```python
from build123d import *

# Parameters (mm, degrees)
BOSS_EXTRUDE1_DEPTH   = 9
BOSS_EXTRUDE1_2_DEPTH = 9
SKETCH1_3_W           = 6
SKETCH1_3_H           = 30
BOSS_EXTRUDE2_DEPTH   = 28
BOSS_EXTRUDE2_2_DEPTH = 28
SKETCH1_4_W           = 4
SKETCH1_4_H           = 7
BOSS_EXTRUDE3_DEPTH   = 40
BOSS_EXTRUDE3_2_DEPTH = 40
BOSS_EXTRUDE3_3_DEPTH = 40
BOSS_EXTRUDE3_4_DEPTH = 40
SKETCH1_5_W           = 10
SKETCH1_5_H           = 3
BOSS_EXTRUDE4_DEPTH   = 35.5
BOSS_EXTRUDE4_2_DEPTH = 35.5
SKETCH1_6_W           = 120
SKETCH1_6_H           = 60
BOSS_EXTRUDE5_DEPTH   = 2
SKETCH1_8_W           = 28.6
SKETCH1_8_H           = 57
SKETCH1_8_W_2         = 22.6
SKETCH1_8_H_2         = 51
BOSS_EXTRUDE6_DEPTH   = 9
SKETCH1_9_W           = 22.6
SKETCH1_9_H           = 0.6
BOSS_EXTRUDE7_DEPTH   = 9
SKETCH2_W             = 6
SKETCH2_H             = 3.75
BOSS_EXTRUDE8_DEPTH   = 13
BOSS_EXTRUDE9_DEPTH   = 3
SKETCH3_5_R           = 1.5
BOSS_EXTRUDE11_DEPTH  = 8
SKETCH4_R             = 4.5
SKETCH4_R_2           = 1.5
BOSS_EXTRUDE13_DEPTH  = 4
SKETCH4_4_R           = 1.5
CUT_EXTRUDE2_DEPTH    = 4
SKETCH5_R             = 4.5
SKETCH5_R_2           = 1.5
BOSS_EXTRUDE14_DEPTH  = 4
SKETCH5_2_R           = 1.5
CUT_EXTRUDE3_DEPTH    = 4
SKETCH7_R             = 4.5
SKETCH7_R_2           = 1.5
BOSS_EXTRUDE15_DEPTH  = 4
SKETCH7_2_R           = 1.5
CUT_EXTRUDE4_DEPTH    = 4
SKETCH8_R             = 4.5
SKETCH8_R_2           = 1.5
BOSS_EXTRUDE16_DEPTH  = 4
SKETCH8_4_R           = 1.5
CUT_EXTRUDE5_DEPTH    = 4


with BuildPart() as part:
    # Sketch1 → Boss-Extrude1 (new body)
    with BuildSketch(Plane(origin=(0, 0, 0), x_dir=(1, 0, 0), z_dir=(0, 1, 0))):
        Polygon((24.7, -0.6), (24.7, 22), (21.7, 22), (21.7, -3.6), (38.3, -3.6), (38.3, 22), (35.3, 22), (35.3, -0.6), align=None)
    extrude(amount=BOSS_EXTRUDE1_DEPTH)



with BuildPart() as body_2:
    # Sketch1 → Boss-Extrude1 2 (new body)
    with BuildSketch(Plane(origin=(0, 0, 0), x_dir=(1, 0, 0), z_dir=(0, 1, 0))):
        Polygon((-35.3, 22), (-38.3, 22), (-38.3, -3.6), (-21.7, -3.6), (-21.7, 22), (-24.7, 22), (-24.7, -0.6), (-35.3, -0.6), align=None)
    extrude(amount=BOSS_EXTRUDE1_2_DEPTH)


with BuildPart() as body_3:
    # Sketch1<3> → Boss-Extrude2 (new body)
    with BuildSketch(Plane(origin=(0, 0, 0), x_dir=(1, 0, 0), z_dir=(0, 1, 0))):
        with Locations((-48, -15)):
            Rectangle(SKETCH1_3_W, SKETCH1_3_H)
    extrude(amount=BOSS_EXTRUDE2_DEPTH)


with BuildPart() as body_4:
    # Sketch1<3> → Boss-Extrude2 2 (new body)
    with BuildSketch(Plane(origin=(0, 0, 0), x_dir=(1, 0, 0), z_dir=(0, 1, 0))):
        with Locations((48, -15)):
            Rectangle(SKETCH1_3_W, SKETCH1_3_H)
    extrude(amount=BOSS_EXTRUDE2_2_DEPTH)


with BuildPart() as body_5:
    # Sketch1<4> → Boss-Extrude3 (new body)
    with BuildSketch(Plane(origin=(0, 0, 0), x_dir=(1, 0, 0), z_dir=(0, 1, 0))):
        with Locations((-51, 33.5)):
            Rectangle(SKETCH1_4_W, SKETCH1_4_H)
    extrude(amount=BOSS_EXTRUDE3_DEPTH)


with BuildPart() as body_6:
    # Sketch1<4> → Boss-Extrude3 2 (new body)
    with BuildSketch(Plane(origin=(0, 0, 0), x_dir=(1, 0, 0), z_dir=(0, 1, 0))):
        with Locations((-9, 33.5)):
            Rectangle(SKETCH1_4_W, SKETCH1_4_H)
    extrude(amount=BOSS_EXTRUDE3_2_DEPTH)


with BuildPart() as body_7:
    # Sketch1<4> → Boss-Extrude3 3 (new body)
    with BuildSketch(Plane(origin=(0, 0, 0), x_dir=(1, 0, 0), z_dir=(0, 1, 0))):
        with Locations((9, 33.5)):
            Rectangle(SKETCH1_4_W, SKETCH1_4_H)
    extrude(amount=BOSS_EXTRUDE3_3_DEPTH)


with BuildPart() as body_8:
    # Sketch1<4> → Boss-Extrude3 4 (new body)
    with BuildSketch(Plane(origin=(0, 0, 0), x_dir=(1, 0, 0), z_dir=(0, 1, 0))):
        with Locations((51, 33.5)):
            Rectangle(SKETCH1_4_W, SKETCH1_4_H)
    extrude(amount=BOSS_EXTRUDE3_4_DEPTH)


with BuildPart() as body_9:
    # Sketch1<5> → Boss-Extrude4 (new body)
    with BuildSketch(Plane(origin=(0, 0, 0), x_dir=(1, 0, 0), z_dir=(0, 1, 0))):
        with Locations((30, 28.5)):
            Rectangle(SKETCH1_5_W, SKETCH1_5_H)
    extrude(amount=BOSS_EXTRUDE4_DEPTH)


with BuildPart() as body_10:
    # Sketch1<5> → Boss-Extrude4 2 (new body)
    with BuildSketch(Plane(origin=(0, 0, 0), x_dir=(1, 0, 0), z_dir=(0, 1, 0))):
        with Locations((-30, 28.5)):
            Rectangle(SKETCH1_5_W, SKETCH1_5_H)
    extrude(amount=BOSS_EXTRUDE4_2_DEPTH)


with BuildPart() as part_1:
    add(part.part)

    add(body_2.part)  # Boss-Extrude5 merges body 2

    add(body_3.part)  # Boss-Extrude5 merges body 3

    add(body_4.part)  # Boss-Extrude5 merges body 4

    add(body_5.part)  # Boss-Extrude5 merges body 5

    add(body_6.part)  # Boss-Extrude5 merges body 6

    add(body_7.part)  # Boss-Extrude5 merges body 7

    add(body_8.part)  # Boss-Extrude5 merges body 8

    add(body_9.part)  # Boss-Extrude5 merges body 9

    add(body_10.part)  # Boss-Extrude5 merges body 10
    # Sketch1<6> → Boss-Extrude5 (add)
    with BuildSketch(Plane(origin=(0, 0, 0), x_dir=(1, 0, 0), z_dir=(0, 1, 0))):
        Rectangle(SKETCH1_6_W, SKETCH1_6_H)
    extrude(amount=BOSS_EXTRUDE5_DEPTH)

    # Sketch1<8> → Boss-Extrude6 (add)
    with BuildSketch(Plane(origin=(0, 0, 0), x_dir=(1, 0, 0), z_dir=(0, 1, 0))):
        Rectangle(SKETCH1_8_W, SKETCH1_8_H)
        Rectangle(SKETCH1_8_W_2, SKETCH1_8_H_2, mode=Mode.SUBTRACT)
    extrude(amount=BOSS_EXTRUDE6_DEPTH)

    # Sketch1<9> → Boss-Extrude7 (add)
    with BuildSketch(Plane(origin=(0, 0, 0), x_dir=(1, 0, 0), z_dir=(0, 1, 0))):
        with Locations((0, 12.9)):
            Rectangle(SKETCH1_9_W, SKETCH1_9_H)
        Rectangle(SKETCH1_9_W, SKETCH1_9_H)
        with Locations((0, -12.9)):
            Rectangle(SKETCH1_9_W, SKETCH1_9_H)
    extrude(amount=BOSS_EXTRUDE7_DEPTH)

    # Sketch2 → Boss-Extrude8 (add)
    with BuildSketch(Plane(origin=(0, 28, 0), x_dir=(1, 0, 0), z_dir=(0, 1, 0))):
        with Locations((-48, -1.875)):
            Rectangle(SKETCH2_W, SKETCH2_H)
        with Locations((-48, -28.125)):
            Rectangle(SKETCH2_W, SKETCH2_H)
        with Locations((48, -1.875)):
            Rectangle(SKETCH2_W, SKETCH2_H)
        with Locations((48, -28.125)):
            Rectangle(SKETCH2_W, SKETCH2_H)
    extrude(amount=BOSS_EXTRUDE8_DEPTH)

    # Sketch3 → Boss-Extrude9 (add)
    with BuildSketch(Plane.XY.offset(-27)):
        with BuildLine():
            ThreePointArc((-31.5, 35.5), (-30, 37), (-28.5, 35.5))
            Line((-28.5, 35.5), (-25, 35.5))
            ThreePointArc((-25, 35.5), (-30, 40.5), (-35, 35.5))
            Line((-35, 35.5), (-31.5, 35.5))
        make_face()
        with BuildLine():
            ThreePointArc((28.5, 35.5), (30, 37), (31.5, 35.5))
            Line((31.5, 35.5), (35, 35.5))
            ThreePointArc((35, 35.5), (30, 40.5), (25, 35.5))
            Line((25, 35.5), (28.5, 35.5))
        make_face()
    extrude(amount=-BOSS_EXTRUDE9_DEPTH)

    # Sketch3<5> → Boss-Extrude11 (add)
    with BuildSketch(Plane.XY.offset(-27)):
        with Locations((-30, 35.5)):
            Circle(SKETCH3_5_R)
        with Locations((30, 35.5)):
            Circle(SKETCH3_5_R)
    extrude(amount=-BOSS_EXTRUDE11_DEPTH)

    # Sketch4 → Boss-Extrude13 (add)
    with BuildSketch(Plane.ZY.offset(53)):
        with Locations((-37, 35.5)):
            Circle(SKETCH4_R)
        with Locations((-37, 35.5)):
            Circle(SKETCH4_R_2, mode=Mode.SUBTRACT)
    extrude(amount=-BOSS_EXTRUDE13_DEPTH)

    # Sketch4<4> → Cut-Extrude2 (cut)
    with BuildSketch(Plane.ZY.offset(53)):
        with Locations((-37, 35.5)):
            Circle(SKETCH4_4_R)
    extrude(amount=-CUT_EXTRUDE2_DEPTH, mode=Mode.SUBTRACT)

    # Sketch5 → Boss-Extrude14 (add)
    with BuildSketch(Plane.ZY.offset(11)):
        with Locations((-37, 35.5)):
            Circle(SKETCH5_R)
        with Locations((-37, 35.5)):
            Circle(SKETCH5_R_2, mode=Mode.SUBTRACT)
    extrude(amount=-BOSS_EXTRUDE14_DEPTH)

    # Sketch5<2> → Cut-Extrude3 (cut)
    with BuildSketch(Plane.ZY.offset(11)):
        with Locations((-37, 35.5)):
            Circle(SKETCH5_2_R)
    extrude(amount=-CUT_EXTRUDE3_DEPTH, mode=Mode.SUBTRACT)

    # Sketch7 → Boss-Extrude15 (add)
    with BuildSketch(Plane.ZY.offset(-7)):
        with Locations((-37, 35.5)):
            Circle(SKETCH7_R)
        with Locations((-37, 35.5)):
            Circle(SKETCH7_R_2, mode=Mode.SUBTRACT)
    extrude(amount=-BOSS_EXTRUDE15_DEPTH)

    # Sketch7<2> → Cut-Extrude4 (cut)
    with BuildSketch(Plane.ZY.offset(-7)):
        with Locations((-37, 35.5)):
            Circle(SKETCH7_2_R)
    extrude(amount=-CUT_EXTRUDE4_DEPTH, mode=Mode.SUBTRACT)

    # Sketch8 → Boss-Extrude16 (add)
    with BuildSketch(Plane.ZY.offset(-49)):
        with Locations((-37, 35.5)):
            Circle(SKETCH8_R)
        with Locations((-37, 35.5)):
            Circle(SKETCH8_R_2, mode=Mode.SUBTRACT)
    extrude(amount=-BOSS_EXTRUDE16_DEPTH)

    # Sketch8<4> → Cut-Extrude5 (cut)
    with BuildSketch(Plane.ZY.offset(-49)):
        with Locations((-37, 35.5)):
            Circle(SKETCH8_4_R)
    extrude(amount=-CUT_EXTRUDE5_DEPTH, mode=Mode.SUBTRACT)


solid = part_1.part
```
Model file for the job. Use its own axes, mm. A direction names the side the tool comes from. Give positions to 0.01 mm unless a question says otherwise; leave off trailing zeros. Loops run counter-clockwise (first coordinate to the right, second up) from the corner with the lowest first, then second, coordinate; pieces in that order, holes last. Notation, with made-up numbers: (78.25, -19) - (127.25, -19) arc R21 cw to (127.25, 18) - close; hole circle Ø1 at (15.25, 0). An arc over 180 degrees is marked (long way). One line per item, written item: value. Start each with the question number.
1. Probe L1, parallel to X at y = 3, z = -35; L2, parallel to X at y = 8, z = 13.5; L3, parallel to X at y = 6, z = -9. List the from-to ranges inside material, lowest first. Write a range as from..to.
2. Slice it at D-D (z = -9.5). List the corners of the cut face in (x, y).
3. Slice it at A-A (y = 24.5). Give the number of separate pieces and of enclosed holes in the cut face, plus the area to 3 significant figures.
4. Slice it at B-B (z = 10). List the corners of the cut face in (x, y).
5. Which spindle directions (+Z, -Z, +X, -X, +Y, -Y) get a long thin tool onto all of the face, cutting with end or side? Do faces 4 (the flat face through (21.7, 5, -9)), 5 (the flat face through (24, 9, -9)), 6 (the flat face through (-48, 34, 3.75)), 7 (the flat face through (-24.7, 5, -11)), 8 (the flat face through (51, 40, -34)). Say none if no direction does.
6. Slice it at C-C (x = -30). List the corners of the cut face in (y, z), plus the area to 4 significant figures.
7. Pin check, flat tips, straight feed: pin 1 (8 mm diameter, centred on y = 14, z = -30.5, fed in from -X); pin 2 (5.5 mm diameter, centred on y = 6, z = -10, fed in from +X); pin 3 (1.5 mm diameter, centred on y = 23, z = -28.5, fed in from -X). Stop position of each tip, or through.
8. Pull direction X, two halves, no side cores. Call faces 1 (the flat face through (0, 5, 13.2)), 2 (the flat face through (-35, 19, -28)), 3 (the flat face through (9, 40, -34)): pulls with the +X half, pulls with the -X half, needs draft (parallel to the pull), parting line crosses it, or undercut.
Solution:
1. L1: x = -53..-49, -11..-7, 7..11, 49..53
1. L2: x = -51..-45, -14.3..-11.3, 11.3..14.3, 45..51
1. L3: x = -38.3..-35.3, -24.7..-21.7, -14.3..-11.3, 11.3..14.3, 21.7..24.7, 35.3..38.3
2. outline: (-60, 0) - (60, 0) - (60, 2) - (38.3, 2) - (38.3, 9) - (35.3, 9) - (35.3, 2) - (24.7, 2) - (24.7, 9) - (21.7, 9) - (21.7, 2) - (14.3, 2) - (14.3, 9) - (11.3, 9) - (11.3, 2) - (-11.3, 2) - (-11.3, 9) - (-14.3, 9) - (-14.3, 2) - (-21.7, 2) - (-21.7, 9) - (-24.7, 9) - (-24.7, 2) - (-35.3, 2) - (-35.3, 9) - (-38.3, 9) - (-38.3, 2) - (-60, 2) - close
3. separate pieces: 8
3. enclosed holes: 0
3. area: 532 mm^2
4. outline: (-60, 0) - (60, 0) - (60, 2) - (51, 2) - (51, 28) - (45, 28) - (45, 2) - (14.3, 2) - (14.3, 9) - (11.3, 9) - (11.3, 2) - (-11.3, 2) - (-11.3, 9) - (-14.3, 9) - (-14.3, 2) - (-45, 2) - (-45, 28) - (-51, 28) - (-51, 2) - (-60, 2) - close
5. face 4: +Z, -Z, +Y
5. face 5: +Z, +Y
5. face 6: +X, -X, +Y
5. face 7: -Z, +Y
5. face 8: -Z, +X, -X, +Y
6. outline: (0, -30) - (34, -30) - (34, -35) - (37, -35) - (37, -30) - (40.5, -30) - (40.5, -27) - (2, -27) - (2, 0.6) - (9, 0.6) - (9, 3.6) - (2, 3.6) - (2, 30) - (0, 30) - close
6. area: 271.5 mm^2
7. pin 1: stops at x = -53
7. pin 2: stops at x = 38.3
7. pin 3: stops at x = -35
8. face 1: undercut
8. face 2: pulls with the -X half
8. face 3: needs draft
